Part model, mm, in its own coordinate system. Face numbers are marked on the shaded views. Round coordinates to 2 decimals unless told otherwise and drop trailing zeros. Order: outer loops, then holes, each group sorted by start corner. A loop starts at its lowest first (then second) coordinate and runs counter-clockwise, first axis right, second up. Notation, with made-up numbers: (7.25, 47.5) -> (22.25, 47.5) arc R22 cw to (22.25, 84.5) -> close; hole circle Ø11 at (47.25, -39.75). An arc over 180 degrees is marked (long way). Return JSON: item names as keys, results as strings. Group by question number.
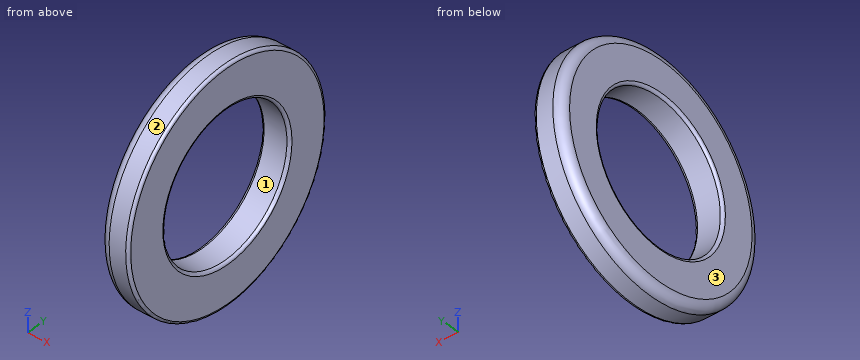
from build123d import *

# Parameters (mm, degrees)
SKETCH1_R           = 6.365
SKETCH1_R_2         = 4
BOSS_EXTRUDE1_DEPTH = 1.57
FILLET1_R           = 0.15
FILLET2_R           = 0.15
FILLET3_R           = 0.5


with BuildPart() as part:
    # Sketch1 → Boss-Extrude1 (new body)
    with BuildSketch(Plane(origin=(0, 0, 0), x_dir=(0, 0, -1), z_dir=(1, 0, 0))):
        Circle(SKETCH1_R)
        Circle(SKETCH1_R_2, mode=Mode.SUBTRACT)
    extrude(amount=BOSS_EXTRUDE1_DEPTH)

    # Fillet1
    fillet1_edges = [part.edges().sort_by_distance(p)[0] for p in [
        (1.57, 0, 6.365),
        (1.57, 0, 4),
    ]]
    fillet(fillet1_edges, radius=FILLET1_R)

    # Fillet2
    fillet2_edges = [part.edges().sort_by_distance(p)[0] for p in [
        (0, 0, 4),
    ]]
    fillet(fillet2_edges, radius=FILLET2_R)

    # Fillet3
    fillet3_edges = [part.edges().sort_by_distance(p)[0] for p in [
        (0, 0, 6.365),
    ]]
    fillet(fillet3_edges, radius=FILLET3_R)


solid = part.part
(1) Mould opens along Z. For the marked faces 1, 2 and 3 say: pulls with the +Z half, pulls with the -Z half, needs draft (parallel to the pull), parting line crosses it, or undercut.
(2) Saw through at A-A, the plane y = 0. List the corners of the cut face in (x, z) (3 decimals), and give its area (3 significant figures).
(3) Probe L1, parallel to Y at x = 0.9, z = 0 (3 decimals); L2, parallel to Z at x = 1.2, y = 0.25; L3, parallel to Z at x = 0.7, y = -2.75. List the from-to ranges inside material, lowest first. Write a range as [from, to].
(4) Pin check, flat tip, straight feed: P1, Ø4, axis at y = 0.5, z = -0.5, coming from the +X side. Stop position of the tip, or through.
(5) Saw through at C-C, the plane x = 0.7. List the corners of the cut face in (y, z) (3 decimals), and give its area (3 significant figures).
Results are:
{
 "1": {"face 1": "undercut", "face 2": "parting line crosses it", "face 3": "needs draft"},
 "2": {"outline": "(0, -5.865) arc R0.5 ccw to (0.5, -6.365) -> (1.42, -6.365) arc R0.15 ccw to (1.57, -6.215) -> (1.57, -4.15) arc R0.15 ccw to (1.42, -4) -> (0.15, -4) arc R0.15 ccw to (0, -4.15) -> close; (0, 4.15) arc R0.15 ccw to (0.15, 4) -> (1.42, 4) arc R0.15 ccw to (1.57, 4.15) -> (1.57, 6.215) arc R0.15 ccw to (1.42, 6.365) -> (0.5, 6.365) arc R0.5 ccw to (0, 5.865) -> close", "area": "7.29 mm^2"},
 "3": {"L1": "y = [-6.365, -4], [4, 6.365]", "L2": "z = [-6.36, -3.99], [3.99, 6.36]", "L3": "z = [-5.74, -2.9], [2.9, 5.74]"},
 "4": {"P1": "passes through"},
 "5": {"outline": "circle Ø12.73 at (0, 0); hole circle Ø8 at (0, 0)", "area": "77.0 mm^2"}
}
